The listing builds one solid part. Answer for the finished solid, in the listing's coordinates (mm). Face numbers are marked on the shaded views. A direction names the side the tool comes from. Round coordinates to 2 decimals unless told otherwise and drop trailing zeros. Write each loop counter-clockwise with the first axis right and the second up, starting at its lowest first coordinate (ties: lowest second). Pieces come first, ordered by that corner, then holes.
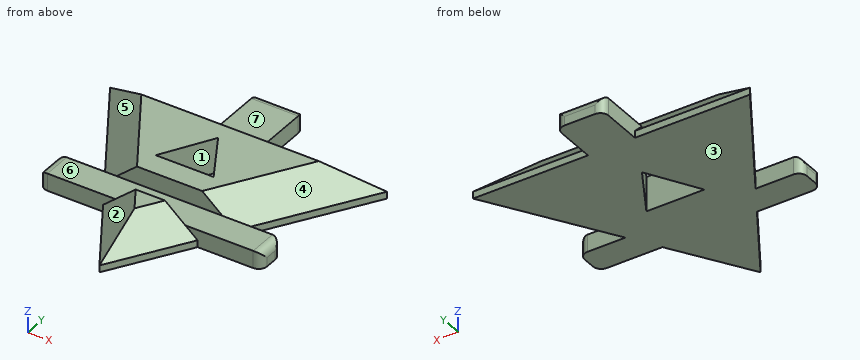
from build123d import *

# Parameters (mm, degrees)
F1_DEPTH     = 3.175
F2_W         = 20.397445187
F2_H         = 2.647349927
F2_W_2       = 4.2995549738
F2_H_2       = 13.8314400401
F3_DEPTH     = 1.5875
F4_W         = 14.3783436368
F4_H         = 2.647349927
F5_DEPTH     = 25.4
F6_T4_DEPTH  = 25.8319450188
F6_T9_DEPTH  = 25.8319450188
F6_T14_DEPTH = 38.4641495789
F6_T19_DEPTH = 38.4641495789
F6_T24_DEPTH = 38.4641495789
F6_T29_DEPTH = 25.8319450188
F6_T34_DEPTH = 25.8319450188
F6_T39_DEPTH = 21.2914590052
F6_T44_DEPTH = 21.2914590052
F6_T49_DEPTH = 21.2914590052
F6_T54_DEPTH = 21.2914590052
F7_R         = 0.762
F9_DEPTH     = 25.4


# Not quite as in the source:
# - a fillet or chamfer that OpenCascade refuses, or shapes differently, is made with other operations: its cross-section is extruded or revolved along the edge and cut away or added


with BuildPart() as f1:
    # F0 (on Top) → F1 (new body)
    with BuildSketch(Plane.XY):
        Polygon((12.7, 7.7934656292), (-12.7, 7.7934656292), (0, -12.7), align=None)
    extrude(amount=F1_DEPTH)

    # F2 (on Top) → F3 (join)
    with BuildSketch(Plane.XY):
        with Locations((0, -4.3830036468)):
            Rectangle(F2_W, F2_H)
        with Locations((0, 5.2467339706)):
            Rectangle(F2_W_2, F2_H_2)
    extrude(amount=F3_DEPTH)

    # F4 (on face) → F5 (cut)
    with BuildSketch(Plane.XY.offset(1.5875)):
        with Locations((-1.2147540241, -4.3830036468)):
            Rectangle(F4_W, F4_H)
    extrude(amount=F5_DEPTH, mode=Mode.SUBTRACT)

    # F6: chamfer of 2.54 on 5 edges, made by hand


with BuildPart() as f6_tool2:
    # F6_s3 → F6_t4 (new body)
    with BuildSketch(Plane(origin=(-10.454367288, 16.8697808418, 0), x_dir=(0, 0, 1), z_dir=(0.5267614317, -0.8500131729, 0))):
        Polygon((0.635, 6.6898701827), (3.175, 4.1498701827), (3.175, 6.6898701827), align=None)
    extrude(amount=F6_T4_DEPTH)

    split(bisect_by=Plane.XZ.offset(3.0593286833), keep=Keep.BOTTOM)


with BuildPart() as f1_1:
    add(f1.part)

    # F6_t1: cut F6_tool2
    add(f6_tool2.part, mode=Mode.SUBTRACT)


with BuildPart() as f6_tool7:
    # F6_s8 → F6_t9 (new body)
    with BuildSketch(Plane(origin=(-10.454367288, 16.8697808418, 0), x_dir=(0, 0, 1), z_dir=(0.5267614317, -0.8500131729, 0))):
        Polygon((0.635, 6.6898701827), (3.175, 4.1498701827), (3.175, 6.6898701827), align=None)
    extrude(amount=F6_T9_DEPTH)

    split(bisect_by=Plane.XZ.offset(5.7066786103), keep=Keep.TOP)


with BuildPart() as f1_2:
    add(f1_1.part)

    # F6_t6: cut F6_tool7
    add(f6_tool7.part, mode=Mode.SUBTRACT)


with BuildPart() as f6_tool12:
    # F6_s13 → F6_t14 (new body)
    with BuildSketch(Plane.YZ.offset(19.2320747894)):
        Polygon((7.7934656292, 0.635), (5.2534656292, 3.175), (7.7934656292, 3.175), align=None)
    extrude(amount=-F6_T14_DEPTH)

    split(bisect_by=Plane.YZ.offset(2.1497774869), keep=Keep.TOP)


with BuildPart() as f1_3:
    add(f1_2.part)

    # F6_t11: cut F6_tool12
    add(f6_tool12.part, mode=Mode.SUBTRACT)


with BuildPart() as f6_tool17:
    # F6_s18 → F6_t19 (new body)
    with BuildSketch(Plane.YZ.offset(19.2320747894)):
        Polygon((7.7934656292, 0.635), (5.2534656292, 3.175), (7.7934656292, 3.175), align=None)
    extrude(amount=-F6_T19_DEPTH)

    split(bisect_by=Plane.XY.offset(1.5875), keep=Keep.TOP)


with BuildPart() as f1_4:
    add(f1_3.part)

    # F6_t16: cut F6_tool17
    add(f6_tool17.part, mode=Mode.SUBTRACT)


with BuildPart() as f6_tool22:
    # F6_s23 → F6_t24 (new body)
    with BuildSketch(Plane.YZ.offset(19.2320747894)):
        Polygon((7.7934656292, 0.635), (5.2534656292, 3.175), (7.7934656292, 3.175), align=None)
    extrude(amount=-F6_T24_DEPTH)

    split(bisect_by=Plane.YZ.offset(-2.1497774869), keep=Keep.BOTTOM)


with BuildPart() as f1_5:
    add(f1_4.part)

    # F6_t21: cut F6_tool22
    add(f6_tool22.part, mode=Mode.SUBTRACT)


with BuildPart() as f6_tool27:
    # F6_s28 → F6_t29 (new body)
    with BuildSketch(Plane(origin=(-3.1529050539, -5.0877127051, 0), x_dir=(0, 0, 1), z_dir=(0.5267614317, 0.8500131729, 0))):
        Polygon((0.635, 6.6898701827), (3.175, 4.1498701827), (3.175, 6.6898701827), align=None)
    extrude(amount=F6_T29_DEPTH)

    split(bisect_by=Plane.XZ.offset(5.7066786103), keep=Keep.TOP)


with BuildPart() as f1_6:
    add(f1_5.part)

    # F6_t26: cut F6_tool27
    add(f6_tool27.part, mode=Mode.SUBTRACT)


with BuildPart() as f6_tool32:
    # F6_s33 → F6_t34 (new body)
    with BuildSketch(Plane(origin=(-3.1529050539, -5.0877127051, 0), x_dir=(0, 0, 1), z_dir=(0.5267614317, 0.8500131729, 0))):
        Polygon((0.635, 6.6898701827), (3.175, 4.1498701827), (3.175, 6.6898701827), align=None)
    extrude(amount=F6_T34_DEPTH)

    split(bisect_by=Plane.XZ.offset(3.0593286833), keep=Keep.BOTTOM)


with BuildPart() as f1_7:
    add(f1_6.part)

    # F6_t31: cut F6_tool32
    add(f6_tool32.part, mode=Mode.SUBTRACT)


with BuildPart() as f6_tool37:
    # F6_s38 → F6_t39 (new body)
    with BuildSketch(Plane(origin=(-9.1273228482, -14.7283840218, 0), x_dir=(0, 0, 1), z_dir=(0.5267614317, 0.8500131729, 0))):
        Polygon((0.635, 6.6898701827), (3.175, 4.1498701827), (3.175, 6.6898701827), align=None)
    extrude(amount=F6_T39_DEPTH)

    split(bisect_by=Plane.XZ.offset(5.7066786103), keep=Keep.TOP)


with BuildPart() as f1_8:
    add(f1_7.part)

    # F6_t36: cut F6_tool37
    add(f6_tool37.part, mode=Mode.SUBTRACT)


with BuildPart() as f6_tool42:
    # F6_s43 → F6_t44 (new body)
    with BuildSketch(Plane(origin=(-9.1273228482, -14.7283840218, 0), x_dir=(0, 0, 1), z_dir=(0.5267614317, 0.8500131729, 0))):
        Polygon((0.635, 6.6898701827), (3.175, 4.1498701827), (3.175, 6.6898701827), align=None)
    extrude(amount=F6_T44_DEPTH)

    split(bisect_by=Plane.XZ.offset(3.0593286833), keep=Keep.BOTTOM)


with BuildPart() as f1_9:
    add(f1_8.part)

    # F6_t41: cut F6_tool42
    add(f6_tool42.part, mode=Mode.SUBTRACT)


with BuildPart() as f6_tool47:
    # F6_s48 → F6_t49 (new body)
    with BuildSketch(Plane(origin=(-2.0881965805, 3.3696366023, 0), x_dir=(0, 0, 1), z_dir=(0.5267614317, -0.8500131729, 0))):
        Polygon((0.635, 6.6898701827), (3.175, 4.1498701827), (3.175, 6.6898701827), align=None)
    extrude(amount=F6_T49_DEPTH)

    split(bisect_by=Plane.XZ.offset(3.0593286833), keep=Keep.BOTTOM)


with BuildPart() as f1_10:
    add(f1_9.part)

    # F6_t46: cut F6_tool47
    add(f6_tool47.part, mode=Mode.SUBTRACT)


with BuildPart() as f6_tool52:
    # F6_s53 → F6_t54 (new body)
    with BuildSketch(Plane(origin=(-2.0881965805, 3.3696366023, 0), x_dir=(0, 0, 1), z_dir=(0.5267614317, -0.8500131729, 0))):
        Polygon((0.635, 6.6898701827), (3.175, 4.1498701827), (3.175, 6.6898701827), align=None)
    extrude(amount=F6_T54_DEPTH)

    split(bisect_by=Plane.XZ.offset(5.7066786103), keep=Keep.TOP)


with BuildPart() as f1_11:
    add(f1_10.part)

    # F6_t51: cut F6_tool52
    add(f6_tool52.part, mode=Mode.SUBTRACT)

    # F7
    f7_edges = [f1_11.edges().sort_by_distance(p)[0] for p in [
        (-2.149777, 12.162454, 0.79375),
        (0, 12.162454, 1.5875),
        (2.149777, 12.162454, 0.79375),
        (-10.198723, -4.383004, 1.5875),
        (-10.198723, -5.706679, 0.79375),
        (-10.198723, -3.059329, 0.79375),
        (10.198723, -3.059329, 0.79375),
        (10.198723, -5.706679, 0.79375),
        (10.198723, -4.383004, 1.5875),
    ]]
    fillet(f7_edges, radius=F7_R)

    # F8 (on face) → F9 (cut)
    with BuildSketch(Plane.XY.offset(3.175)):
        Polygon((-2.6549665111, -0.989894278), (0, -0.989894278), (2.6549665111, -0.989894278), (0, 3.6086426117), align=None)
    extrude(amount=-F9_DEPTH, mode=Mode.SUBTRACT)


solid = f1_11.part
1. Straight lines are drawn through the part: line 1 along Y through (x, z) = (0.25, 2.5); line 2 along Z through (x, y) = (-8.25, -3.5); line 3 along Y through (x, z) = (0.25, 2). For each, find the intervals that lie inside material, in ascending order.
Geometry says:
line 1: y = -8.76 to -5.71, -3.06 to -0.99, 3.18 to 5.93
line 2: z = 0 to 1.59
line 3: y = -9.71 to -5.71, -3.06 to -0.99, 3.18 to 6.43
2. Section D-D on y = -4.5 is taken. Determine the outline of the cut face in (x, z).
Geometry says:
outline: (-10.2, 0) - (10.2, 0) - (10.2, 0.83) arc R0.76 ccw to (9.44, 1.59) - (-9.44, 1.59) arc R0.76 ccw to (-10.2, 0.83) - close
3. Section B-B on y = 1.5 is taken. Determine the outline of the cut face in (x, z) (3 decimals), plus the area to 3 significant figures.
Geometry says:
outline: (-8.8, 0) - (-1.217, 0) - (-1.217, 3.175) - (-5.812, 3.175) - (-8.8, 0.635) - close; (1.217, 0) - (8.8, 0) - (8.8, 0.635) - (5.812, 3.175) - (1.217, 3.175) - close
area: 40.6 mm2
4. For a pull along Y with two mould halves and no side action, classify the marked faces 1, 2 and 3 as released by +Y, released by -Y, zero draft, split by the parting line, or undercut.
Geometry says:
face 1: undercut
face 2: released by -Y
face 3: zero draft
5. A tool of negligible diameter and unlimited length cuts with its end or side. For the marked faces 4, 5, 6 and 7, from which of +Z, -Z, +X, -X, +Y, -Y can it reach the whole face along a straight path? Write none if from no direction.
Geometry says:
face 4: +Z, +X
face 5: +Z, -X
face 6: +Z, +X, -X
face 7: +Z, +X, -X, +Y
6. Given pin 1 (1 mm diameter, centred on x = -10, y = -3.5, fed in from +Z); pin 2 (0.8 mm diameter, centred on x = -7, z = 1, fed in from +Y); pin 3 (1.7 mm diameter, centred on x = -2, z = 2.5, fed in from -Y), each flat-ended and moving along its own axis, determine where each tip first touches the part or whether it passes through.
Geometry says:
pin 1: stops at z = 1.58
pin 2: stops at y = 7.79
pin 3: stops at y = -8.05
7. Section A-A on z = 2.2 is taken. Determine the outline of the cut face in (x, y), plus the area to 3 significant figures.
Geometry says:
outline: (-9.89, 6.23) - (-4.13, -3.06) - (4.13, -3.06) - (9.89, 6.23) - close; (-2.49, -5.71) - (0, -9.73) - (2.49, -5.71) - close; hole (-2.65, -0.99) - (2.65, -0.99) - (0, 3.61) - close
area: 128 mm2
8. Section C-C on x = 1.75 is taken. Determine the outline of the cut face in (y, z) (1 decimal), plus the area to 3 significant figures.
Geometry says:
outline: (-9.9, 0) - (-1, 0) - (-1, 3.2) - (-3.1, 3.2) - (-3.1, 1.6) - (-5.7, 1.6) - (-5.7, 2.8) - (-9.9, 0.6) - close; (0.6, 0) - (12.1, 0) - (12.1, 1.2) arc R0.8 ccw to (11.4, 1.6) - (6.8, 1.6) - (5.3, 3.2) - (0.6, 3.2) - close
area: 44.9 mm2
